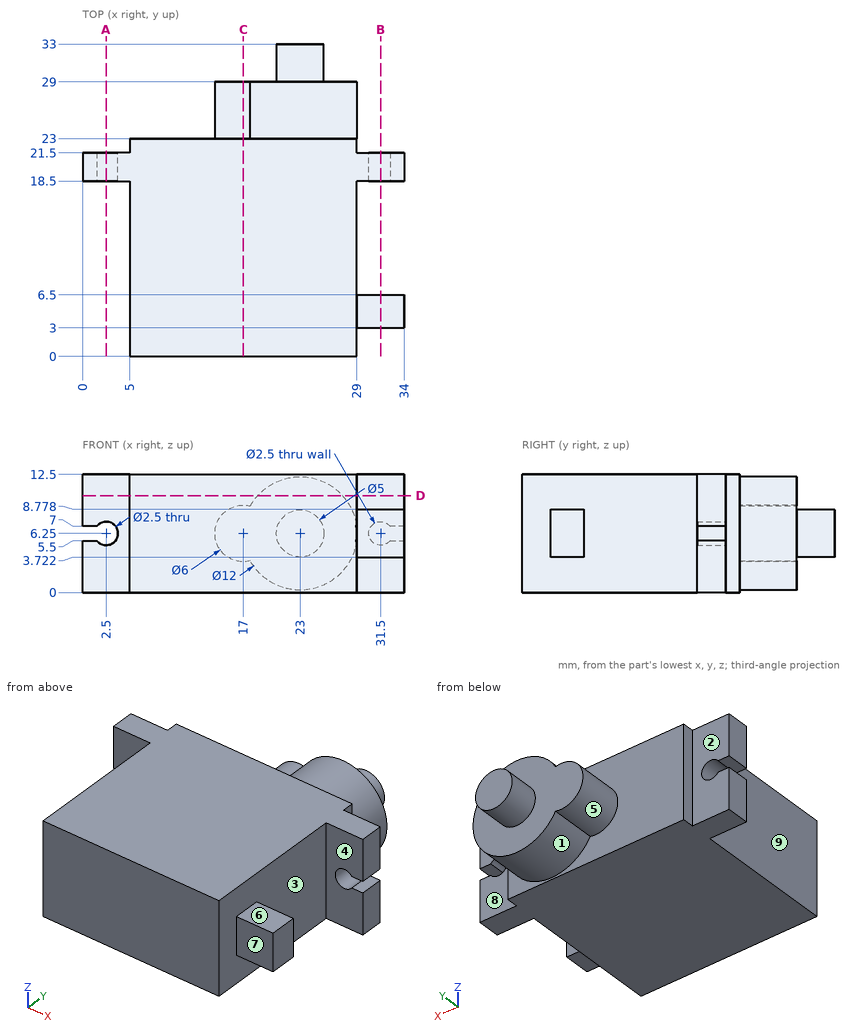
The drawing under review shows one solid part. Ordinate dimensions are in mm from its lowest x, y, z. A direction names the side the tool comes from. Give positions to 0.01 mm unless a question says otherwise; leave off trailing zeros. Order: outer loops, then holes, each group sorted by start corner. A loop starts at its lowest first (then second) coordinate and runs counter-clockwise, first axis right, second up. Notation, with made-up numbers: (86, 42) -> (94, 42) arc R27 ccw to (94, 68) -> close; hole circle Ø7 at (-25.75, 1.5). An arc over 180 degrees is marked (long way). Write item = value, one per line.
1) We need section C-C, the plane x = 17. Give the boundary of the cut face in (y, z).
Findings:
outline = (0, 0) -> (23, 0) -> (23, 3.25) -> (29, 3.25) -> (29, 9.25) -> (23, 9.25) -> (23, 12.5) -> (0, 12.5) -> close
2) To check wall thickness, follow L1, parallel to Z at x = 2.5, y = 19.8; L2, parallel to Y at x = 18.5, z = 8; L3, parallel to X at y = 17.5, z = 4.25. State the ranges of each line that lie inside material, in increasing order. Write a range as from..to.
Findings:
L1 = 0..5, 7.5..12.5
L2 = 0..29
L3 = 5..29
3) We need section B-B, the plane x = 31.5. Give the boundary of the cut face in (y, z).
Findings:
outline = (3, 3.72) -> (6.5, 3.72) -> (6.5, 8.78) -> (3, 8.78) -> close; (18.5, 0) -> (21.5, 0) -> (21.5, 5) -> (18.5, 5) -> close; (18.5, 7.5) -> (21.5, 7.5) -> (21.5, 12.5) -> (18.5, 12.5) -> close
4) We need section D-D, the plane z = 10.25. Give the boundary of the cut face in (x, y), and give its area (3 significant figures).
Findings:
outline = (0, 18.5) -> (5, 18.5) -> (5, 0) -> (29, 0) -> (29, 18.5) -> (34, 18.5) -> (34, 21.5) -> (29, 21.5) -> (29, 23) -> (27.47, 23) -> (27.47, 29) -> (18.53, 29) -> (18.53, 23) -> (5, 23) -> (5, 21.5) -> (0, 21.5) -> close
area = 636 mm^2
5) Draft analysis for pull direction Y (two halves, no side actions). For the marked faces 1, 2, 3 and 4, state which applies: pulls with the +Y half, pulls with the -Y half, needs draft (parallel to the pull), parting line crosses it, or undercut.
Findings:
face_1 = needs draft
face_2 = pulls with the +Y half
face_3 = undercut
face_4 = undercut
6) For the marked faces 5, 6, 7, 8 and 9, list the 3-axis set-ups (+Z, -Z, +X, -X, +Y, -Y) from which the entire face can be reached by the end or side of a thin tool; tool diameter is ignored.
Findings:
face_5 = +Y
face_6 = +Z, +X, -Y
face_7 = +Z, -Z, +X, -Y
face_8 = +Z, -Z, +X, +Y
face_9 = +Z, -Z, -X, -Y
7) Insertion check: pin 1 (4 mm diameter, centred on y = 11.5, z = 4.5, fed in from -X); pin 2 (2.5 mm diameter, centred on x = 30.5, z = 9, fed in from +Y); pin 3 (4 mm diameter, centred on x = 32, z = 6.5, fed in from -Y). Each pin has a flat end and moves straight along its axis. Give the tip position at first contact, or say it passes through.
Findings:
pin_1 = 5
pin_2 = 21.5
pin_3 = 3
8) We need section A-A, the plane x = 2.5. Give the boundary of the cut face in (y, z), and give its area (3 significant figures).
Findings:
outline = (18.5, 0) -> (21.5, 0) -> (21.5, 5) -> (18.5, 5) -> close; (18.5, 7.5) -> (21.5, 7.5) -> (21.5, 12.5) -> (18.5, 12.5) -> close
area = 30.0 mm^2
